Check sheet for the modelled part. Datum: model origin and axes. Units: mm. Face numbers are marked on the shaded views. Round coordinates to 2 decimals unless told otherwise and drop trailing zeros. Loops run counter-clockwise (first coordinate to the right, second up) from the corner with the lowest first, then second, coordinate; pieces in that order, holes last. Notation, with made-up numbers: (85.25, 29.25) - (117.25, 29.25) arc R27 cw to (117.25, 50.25) - close; hole circle Ø11 at (6, -3.75). An arc over 180 degrees is marked (long way). Put each result on its own line as item: value. Start each with the question number.
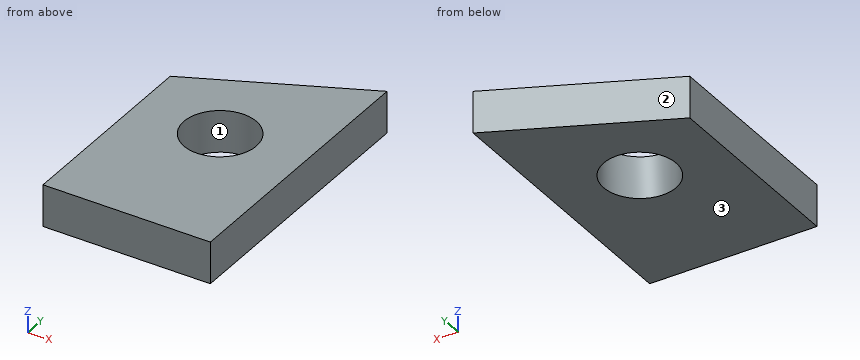
```python
from build123d import *

# Parameters (mm, degrees)
SKETCH2_W           = 12.7
SKETCH2_H           = 3.175
BOSS_EXTRUDE1_DEPTH = 63.5
CUT_EXTRUDE1_REACH  = 66.835
SKETCH3_R           = 2.75


with BuildPart() as part:
    # Sketch2 → Boss-Extrude1 (new body)
    with BuildSketch(Plane(origin=(0, 0, 0), x_dir=(1, 0, 0), z_dir=(0, 1, 0))):
        with Locations((6.35, -1.5875)):
            Rectangle(SKETCH2_W, SKETCH2_H)
    extrude(amount=BOSS_EXTRUDE1_DEPTH)

    # Sketch3 → Cut-Extrude1 (cut, up to next)
    with BuildSketch(Plane(origin=(0, 0, 3.175), x_dir=(-1, 0, 0), z_dir=(0, 0, -1)), mode=Mode.PRIVATE) as cut_extrude1_sk1:
        with Locations(Location((-6.35, 11.197261172, 0), (0, 0, 180))):
            Circle(SKETCH3_R)
    cut_extrude1_tool1 = extrude(cut_extrude1_sk1.sketch, amount=CUT_EXTRUDE1_REACH, mode=Mode.PRIVATE) & part.part
    # Sketch3 → Cut-Extrude1 (cut, up to next)
    with BuildSketch(Plane(origin=(0, 0, 3.175), x_dir=(-1, 0, 0), z_dir=(0, 0, -1)), mode=Mode.PRIVATE) as cut_extrude1_sk2:
        Polygon((-12.7, 21.164764587), (0, 15.242657328), (0, 63.5), (-12.7, 63.5), align=None)
    cut_extrude1_tool2 = extrude(cut_extrude1_sk2.sketch, amount=CUT_EXTRUDE1_REACH, mode=Mode.PRIVATE) & part.part
    add(cut_extrude1_tool1.solids().sort_by_distance((6.35, 11.197261, 3.175))[0], mode=Mode.SUBTRACT)
    add(cut_extrude1_tool2.solids().sort_by_distance((6.211632, 40.819594, 3.175))[0], mode=Mode.SUBTRACT)


solid = part.part
```
Q1. Cross-section at A-A on x = 6.35. Enter the section's corners in (y, z) (3 decimals), and give its area (3 significant figures).
Q2. Material ranges on line 1 (X direction, y = 12, z = 1.15); line 2 (X direction, y = 13.5, z = 1.6); line 3 (Y direction, x = 7.75, z = 2.55), recorded low to high. Write a range as from..to.
Q3. Cross-section at D-D on x = 11.25. Enter the section's corners in (y, z) (3 decimals), and give its area (3 significant figures).
Q4. Draft check along Y on the marked faces 1, 2 and 3. Enter one of: +Y half, -Y half, draft (parallel to the pull), parting line (faces both ways), or undercut.
Q5. Cross-section at C-C on z = 1.8. Enter the section's corners in (x, y).
Q6. Cross-section at B-B on y = 12.5. Enter the section's corners in (x, z) (3 decimals).
Q7. Depth check by flat-ended pin: pin 1 Ø4.5 at (x, y) = (6.35, 11.2) entering from -Z. Enter the tip coordinate at first touch or a pass-through.
Answer list:
1. outline: (0, 0) - (8.447, 0) - (8.447, 3.175) - (0, 3.175) - close; (13.947, 0) - (18.204, 0) - (18.204, 3.175) - (13.947, 3.175) - close
1. area: 40.3 mm2
2. line 1: x = 0..3.72, 8.98..12.7
2. line 2: x = 0..4.85, 7.85..12.7
2. line 3: y = 0..8.83, 13.56..18.86
3. outline: (0, 0) - (20.489, 0) - (20.489, 3.175) - (0, 3.175) - close
3. area: 65.1 mm2
4. face 1: undercut
4. face 2: +Y half
4. face 3: draft
5. outline: (0, 0) - (12.7, 0) - (12.7, 21.16) - (0, 15.24) - close; hole circle Ø5.5 at (6.35, 11.2)
6. outline: (0, 0) - (3.928, 0) - (3.928, 3.175) - (0, 3.175) - close; (8.772, 0) - (12.7, 0) - (12.7, 3.175) - (8.772, 3.175) - close
7. pin 1: passes through
